Geometry: see drawing. Coordinates: mm, zero at the bounding-box minimum. Round coordinates to 2 decimals unless told otherwise and drop trailing zeros. Write each loop counter-clockwise with the first axis right and the second up, starting at its lowest first coordinate (ties: lowest second). Pieces come first, ordered by that corner, then holes.
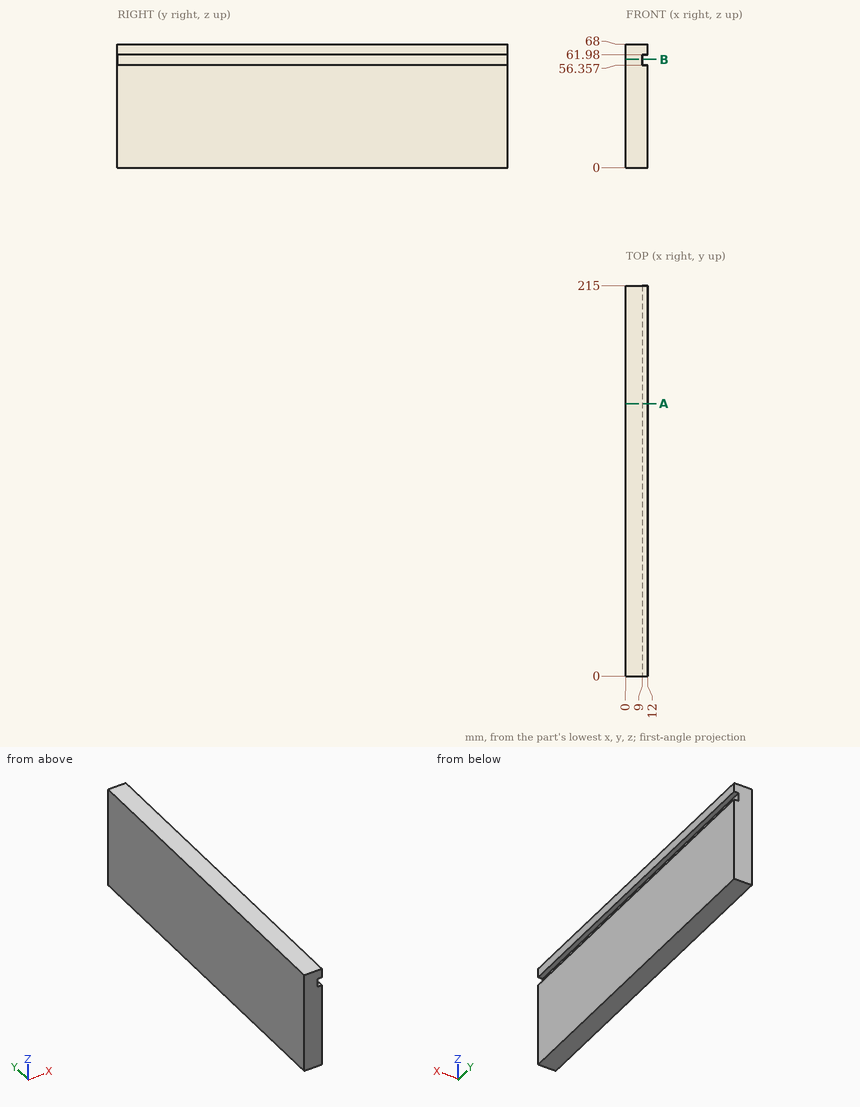
1) Material intervals for line 1 (Z direction, x = 9.75, y = 160.5); line 2 (X direction, y = 179, z = 61.5), sorted ascending.
Taken from the geometry:
line 1: z = 0 to 56.36, 61.98 to 68
line 2: x = 0 to 9
2) Section query B-B on z = 59.5. Return the cut outline in (x, y).
Taken from the geometry:
outline: (0, 0) - (9, 0) - (9, 215) - (0, 215) - close
3) Section query A-A on y = 150. Return the cut outline in (x, z), then the cut area to 3 significant figures.
Taken from the geometry:
outline: (0, 0) - (12, 0) - (12, 56.36) - (9, 56.36) - (9, 61.98) - (12, 61.98) - (12, 68) - (0, 68) - close
area: 799 mm2
